Part model, mm, in its own coordinate system. Face numbers are marked on the shaded views. Give positions to 0.01 mm unless a question says otherwise; leave off trailing zeros. Order: outer loops, then holes, each group sorted by start corner. A loop starts at its lowest first (then second) coordinate and runs counter-clockwise, first axis right, second up. Notation, with made-up numbers: (87, 9) -> (140, 9) arc R31 ccw to (140, 42) -> close; hole circle Ø8 at (38.5, -27). An arc over 180 degrees is marked (long way). Write item = value, one per line. Start each with the question number.
Item 1: Band-saw the part on B-B on y = -24.5. Write the cut outline in (x, z) (3 decimals), plus the area to 3 significant figures.
Item 2: Flat gauge pins, fed straight in: P1, Ø4, axis at x = -20, y = -22.5, coming from the +Z side; P2, Ø8, axis at x = -19, y = -9.5, coming from the -Z side. Where does each tip first touch, or does it go through?
Item 3: Band-saw the part on C-C on x = 5.5. Write the cut outline in (y, z) (3 decimals).
Item 4: Pull direction Y, two halves, no side cores. Call the marked faces 1, 2, 3 and 4: +Y half, -Y half, draft (parallel to the pull), parting line (faces both ways), or undercut.
Item 5: Band-saw the part on D-D on y = -40. Write the cut outline in (x, z) (3 decimals).
Item 6: Drill centre lines: line 1 along Z through (x, y) = (4, -19); line 2 along Y through (x, z) = (18, -20); line 3 along Y through (x, z) = (5.5, 19). Where is each one in solid material? Low to high.
Item 7: Band-saw the part on A-A on z = -16. Write the cut outline in (x, y) (3 decimals).
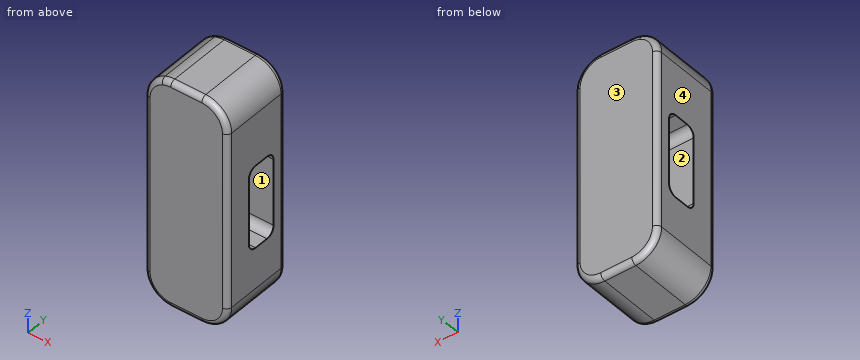
```python
from build123d import *

# Parameters (mm, degrees)
F1_DEPTH = 44.45
F3_DEPTH = 50.801
F4_R     = 3.175


with BuildPart() as f1:
    # F0 (on Front) → F1 (new body)
    with BuildSketch(Plane.XZ):
        with BuildLine():
            ThreePointArc((25.4, 53.975), (20.75032, 65.20032), (9.525, 69.85))
            Line((9.525, 69.85), (-9.525, 69.85))
            ThreePointArc((-9.525, 69.85), (-12.542667, 69.560548), (-15.45029, 68.702748))
            ThreePointArc((-15.45029, 68.702748), (-22.679459, 62.861834), (-25.4, 53.975))
            Line((-25.4, 53.975), (-25.4, -53.975))
            ThreePointArc((-25.4, -53.975), (-20.75032, -65.20032), (-9.525, -69.85))
            Line((-9.525, -69.85), (9.525, -69.85))
            ThreePointArc((9.525, -69.85), (20.75032, -65.20032), (25.4, -53.975))
            Line((25.4, -53.975), (25.4, 53.975))
        make_face()
    extrude(amount=F1_DEPTH)

    # F2 (on face) → F3 (cut, through all)
    with BuildSketch(Plane.YZ.offset(25.4)):
        with BuildLine():
            Line((-13.961844, 22.020357), (-22.851844, 22.020357))
            ThreePointArc((-22.851844, 22.020357), (-26.443946, 20.53246), (-27.931844, 16.940357))
            Line((-27.931844, 16.940357), (-27.931844, -23.699643))
            ThreePointArc((-27.931844, -23.699643), (-26.443946, -27.291745), (-22.851844, -28.779643))
            Line((-22.851844, -28.779643), (-13.961844, -28.779643))
            ThreePointArc((-13.961844, -28.779643), (-10.369742, -27.291745), (-8.881844, -23.699643))
            Line((-8.881844, -23.699643), (-8.881844, 16.940357))
            ThreePointArc((-8.881844, 16.940357), (-10.369742, 20.53246), (-13.961844, 22.020357))
        make_face()
    extrude(amount=-F3_DEPTH, mode=Mode.SUBTRACT)

    # F4
    f4_edges = [f1.edges().sort_by_distance(p)[0] for p in [
        (0, -44.45, 69.85),
        (0, 0, 69.85),
    ]]
    fillet(f4_edges, radius=F4_R)


solid = f1.part
```
Values found:
q1.outline = (-25.4, -53.975) arc R15.875 ccw to (-9.525, -69.85) -> (9.525, -69.85) arc R15.875 ccw to (25.4, -53.975) -> (25.4, -28.505) -> (-25.4, -28.505) -> close; (-25.4, 21.746) -> (25.4, 21.746) -> (25.4, 53.975) arc R15.875 ccw to (9.525, 69.85) -> (-9.525, 69.85) arc R15.875 ccw to (-15.45, 68.703) arc R15.875 ccw to (-25.4, 53.975) -> close
q1.area = 4,330 mm^2
q2.P1 = 67.4
q2.P2 = -68.88
q3.outline = (-44.45, -66.675) arc R3.175 ccw to (-41.275, -69.85) -> (-3.175, -69.85) arc R3.175 ccw to (0, -66.675) -> (0, 66.675) arc R3.175 ccw to (-3.175, 69.85) -> (-41.275, 69.85) arc R3.175 ccw to (-44.45, 66.675) -> close; hole (-27.932, -23.7) arc R5.08 ccw to (-22.852, -28.78) -> (-13.962, -28.78) arc R5.08 ccw to (-8.882, -23.7) -> (-8.882, 16.94) arc R5.08 ccw to (-13.962, 22.02) -> (-22.852, 22.02) arc R5.08 ccw to (-27.932, 16.94) -> close
q4.face_1 = undercut
q4.face_2 = undercut
q4.face_3 = +Y half
q4.face_4 = draft
q5.outline = (-25.4, -53.975) arc R15.875 ccw to (-9.525, -69.85) -> (9.525, -69.85) arc R15.875 ccw to (25.4, -53.975) -> (25.4, 53.975) arc R15.875 ccw to (9.525, 69.85) -> (-9.525, 69.85) arc R15.875 ccw to (-15.45, 68.703) arc R15.875 ccw to (-25.4, 53.975) -> close
q6.line_1 = -69.85 to -28.78, 22.02 to 69.85
q6.line_2 = -44.45 to -27.93, -8.88 to 0
q6.line_3 = -44.45 to -27.5, -9.32 to 0
q7.outline = (-25.4, -41.275) arc R3.175 ccw to (-22.225, -44.45) -> (22.225, -44.45) arc R3.175 ccw to (25.4, -41.275) -> (25.4, -27.932) -> (-25.4, -27.932) -> close; (-25.4, -8.882) -> (25.4, -8.882) -> (25.4, -3.175) arc R3.175 ccw to (22.225, 0) -> (-22.225, 0) arc R3.175 ccw to (-25.4, -3.175) -> close
